```python
from build123d import *

# Parameters (mm, degrees)
F0_R     = 0.625
F1_DEPTH = 4
F2_R     = 1


with BuildPart() as f1:
    # F0 (on Top) → F1 (new body)
    with BuildSketch(Plane.XY):
        with BuildLine():
            ThreePointArc((13.774977, -2.5), (-14, 0), (13.774977, 2.5))
            Line((13.774977, 2.5), (16.309506, 2.5))
            ThreePointArc((16.309506, 2.5), (-16.5, 0), (16.309506, -2.5))
            Line((16.309506, -2.5), (13.774977, -2.5))
        make_face()
        with Locations((14.645819, -4.25)):
            Circle(F0_R, mode=Mode.SUBTRACT)
        with Locations((14.645819, 4.25)):
            Circle(F0_R, mode=Mode.SUBTRACT)
    extrude(amount=F1_DEPTH)

    # F2
    f2_edges = [f1.edges().sort_by_distance(p)[0] for p in [
        (16.309506, 2.5, 2),
        (16.309506, -2.5, 2),
    ]]
    fillet(f2_edges, radius=F2_R)


solid = f1.part
```
The listing builds one solid part. Answer for the finished solid, in the listing's coordinates (mm). A direction names the side the tool comes from. Coordinates: 2 decimals unless noted, no trailing zeros. Loops run counter-clockwise (first coordinate to the right, second up) from the corner with the lowest first, then second, coordinate; pieces in that order, holes last. Notation, with made-up numbers: (3.25, -33) - (47.25, -33) arc R15 ccw to (47.25, -6) - close; hole circle Ø6 at (64.25, 85). An arc over 180 degrees is marked (long way). Use a Markdown table: item, result. Add a question column.
1) The part is cut by section C-C, the plane z = 3.2. Give the vertices of the cut face in (x, y) (3 decimals), and give its area (3 significant figures).
2) The part is cut by section D-D, the plane y = 4.25. Give the vertices of the cut face in (x, z), and give its area (3 significant figures).
3) Given pin 1 (2 mm diameter, centred on x = 14.65, y = -4.25, fed in from +Z); pin 2 (1 mm diameter, centred on y = 12.5, z = 1.5, fed in from +X); pin 3 (1.5 mm diameter, centred on y = -7, z = 1, fed in from +X), each flat-ended and moving along its own axis, determine where each tip first touches the part or whether it passes through.
4) For faces 1 (the cylindrical face through (14.02, -4.22, 1.97)), 2 (the flat face through (14, 2.5, 2)), determine the directions among +Z, -Z, +X, -X, +Y, -Y from which every point of the face is accessible in a straight line to the end or side of a thin tool.
5) The part is cut by section A-A, the plane x = 0. Give the vertices of the cut face in (y, z), and give its area (3 significant figures).
6) The part is cut by section B-B, the plane y = -12. Give the vertices of the cut face in (x, z), and give its area (3 significant figures).
7) Find the intervals of material crossed by line 1 (Y direction, x = 12, z = 3.7); line 2 (Y direction, x = -2, z = 1.05); line 3 (X direction, y = -8, z = 2.8), in increasing order.
8) The mould has two halves that part along Y. Classify faces 3 (the cylindrical face through (-16.486, 0.673, 1.972)), 4 (the flat face through (-14, -4, 0)), 5 (the cylindrical face through (14.02, 4.28, 1.97)): released by +Y, released by -Y, zero draft, split by the parting line, or undercut.
Here are the results:
| question | item | result |
|---|---|---|
| 1 | outline | (13.775, -2.5) arc R14 cw (long way) to (13.775, 2.5) - (15.1, 2.5) arc R1 ccw to (16.074, 3.726) arc R16.5 ccw (long way) to (16.074, -3.726) arc R1 ccw to (15.1, -2.5) - close; hole circle Ø1.25 at (14.646, -4.25); hole circle Ø1.25 at (14.646, 4.25) |
| 1 | area | 224 mm^2 |
| 2 | outline | (-15.94, 0) - (-13.34, 0) - (-13.34, 4) - (-15.94, 4) - close; (13.34, 0) - (14.02, 0) - (14.02, 4) - (13.34, 4) - close; (15.27, 0) - (15.94, 0) - (15.94, 4) - (15.27, 4) - close |
| 2 | area | 15.8 mm^2 |
| 3 | pin 1 | stops at z = 4 |
| 3 | pin 2 | stops at x = 11.32 |
| 3 | pin 3 | stops at x = 15.27 |
| 4 | face 1 | +Z, -Z |
| 4 | face 2 | +Z, -Z, +X |
| 5 | outline | (-16.5, 0) - (-14, 0) - (-14, 4) - (-16.5, 4) - close; (14, 0) - (16.5, 0) - (16.5, 4) - (14, 4) - close |
| 5 | area | 20.0 mm^2 |
| 6 | outline | (-11.32, 0) - (-7.21, 0) - (-7.21, 4) - (-11.32, 4) - close; (7.21, 0) - (11.32, 0) - (11.32, 4) - (7.21, 4) - close |
| 6 | area | 32.9 mm^2 |
| 7 | line 1 | y = -11.32 to -7.21, 7.21 to 11.32 |
| 7 | line 2 | y = -16.38 to -13.86, 13.86 to 16.38 |
| 7 | line 3 | x = -14.43 to -11.49, 11.49 to 14.43 |
| 8 | face 3 | split by the parting line |
| 8 | face 4 | zero draft |
| 8 | face 5 | undercut |
